Part model, mm, in its own coordinate system. A direction names the side the tool comes from. Give positions to 0.01 mm unless a question says otherwise; leave off trailing zeros. Write each loop counter-clockwise with the first axis right and the second up, starting at its lowest first coordinate (ties: lowest second). Pieces come first, ordered by that corner, then holes.
Autodesk Fusion 360 part; units mm, degrees
sketch "Sketch1" plane through (0, 0, 0) normal (0, 0, 1) x (1, 0, 0)
  line L0 (-50.6234, 49.3431) -> (-3.198, -7.4541)
  line L1 (-2.0113, -7.5) -> (224.0597, -7.5)
  line L2 (-30.2635, 80.5455) -> (225.8084, 7.442)
  line L3 (218.275, -2.7029) -> (218.4394, -2.7498)
  arc A0 (225, -2.55) -> (225, 2.55) centre (225, 0) ccw
  arc A1 (224.0597, -7.5) -> (225.8084, 7.442) centre (224.0646, 0.0728) ccw
  arc A2 (-3.198, -7.4541) -> (-2.0113, -7.5) centre (-2.3159, -0.0062) ccw
  arc A3 (-30.2635, 80.5455) -> (-50.6234, 49.3431) centre (-35.6165, 61.7946) ccw
  circle A4 centre (-35.6165, 61.7946) radius 19.5
  line L4 (55, 15) -> (4.1872, -7.5)
  line L5 (-9.5564, 74.634) -> (40, 40)
  line L6 (-10.2571, 1) -> (-10.2571, 29.4154)
  line L7 (-10.2571, 29.4154) -> (-41.41, 38.3089)
  circle A5 centre (220, 0) radius 2.65
  circle A6 centre (-2.3159, -0.0062) radius 2.65
  circle A7 centre (-35.6165, 61.7946) radius 6.25
  circle A8 centre (-35.6165, 61.7946) radius 18.5
  line L8 (5, 35) -> (20, 35)
  line L9 (20, 35) -> (20, 20)
  line L10 (20, 20) -> (5, 20)
  line L11 (5, 20) -> (5, 35)
  line L12 (130, 20) -> (145, 20)
  line L13 (145, 20) -> (145, 5)
  line L14 (145, 5) -> (130, 5)
  line L15 (130, 5) -> (130, 20)
  circle A9 centre (-20.1665, 61.7946) radius 1.55
  circle A10 centre (-27.8915, 75.1747) radius 1.55
  circle A11 centre (-43.3415, 75.1747) radius 1.55
  circle A12 centre (-51.0665, 61.7946) radius 1.55
  circle A13 centre (-43.3415, 48.4145) radius 1.55
  circle A14 centre (-27.8915, 48.4145) radius 1.55
  circle A15 centre (108.8421, -0.0031) radius 2.65
  line L16 (97.1136, -7.5) -> (55, 15)
  line L17 (150.0703, -7.5) -> (179.7021, 5.621)
  line L18 (179.7021, 5.621) -> (204.2609, -7.5)
  line L19 (40, 40) -> (170.5146, 23.2273)
  circle A16 centre (12.5, 27.5) radius 2.65
  circle A17 centre (137.5, 12.5) radius 2.65
  dimension "d10" = 5.1
  dimension "d44" = 39
  dimension "d49" = 5.3
  dimension "d50" = 5.3
  dimension "d66" = 12.5
  dimension "d67" = 37
  dimension "d114" = 3.1
  dimension "d116" = 360
  dimension "d135" = 5.3
  dimension "d140" = 5.3
  dimension "d141" = 5.3
extrude "Extrude24" add sketch "Sketch1" along normal blind 3 contours L0 L1 L2 A1 A2 A4 L4 L5 L6 L7 L16 L17 L18 L19 | A3 A4 | A8 | L8 L9 L10 L11 | L12 L13 L14 L15 | A16 | A17
extrude "Extrude25" add sketch "Sketch1" along normal blind 21.5 contours L8 L9 L10 L11 | L12 L13 L14 L15 | A16 | A17
extrude "Extrude26" cut sketch "Sketch1" along normal blind 22 contours A16 | A17
fillet "Fillet14" radius 5 1 edges at (-41.41, 38.3089, 1.5)
fillet "Fillet15" radius 10 1 edges at (-10.2571, 29.4154, 1.5)
fillet "Fillet16" radius 5 1 edges at (-10.2571, 1, 1.5)
fillet "Fillet17" radius 10 1 edges at (55, 15, 1.5)
fillet "Fillet18" radius 5 1 edges at (97.1136, -7.5, 1.5)
fillet "Fillet19" radius 5 1 edges at (150.0703, -7.5, 1.5)
fillet "Fillet20" radius 10 1 edges at (179.7021, 5.621, 1.5)
fillet "Fillet21" radius 5 1 edges at (204.2609, -7.5, 1.5)
fillet "Fillet22" radius 10 1 edges at (170.5146, 23.2273, 1.5)
fillet "Fillet23" radius 10 1 edges at (40, 40, 1.5)
fillet "Fillet24" radius 5 1 edges at (-9.5564, 74.634, 1.5)
sketch "Sketch4" plane through (0, 0, 3) normal (0, 0, 1) x (-1, 0, 0)
  arc A0 (8.87, -74.1543) -> (10.3617, -74.8639) centre (11.7343, -70.056) ccw
  line L0 (10.3617, -74.8639) -> (30.2635, -80.5455)
  arc A1 (30.2635, -80.5455) -> (50.6234, -49.3431) centre (35.6165, -61.7946) ccw
  line L1 (50.6234, -49.3431) -> (42.396, -39.4898)
  arc A2 (42.396, -39.4898) -> (39.9306, -37.8866) centre (38.558, -42.6945) ccw
  line L2 (39.9306, -37.8866) -> (17.512, -31.4865)
  arc A3 (10.2571, -21.8707) -> (17.512, -31.4865) centre (20.2571, -21.8707) ccw
  line L3 (10.2571, -21.8707) -> (10.2571, -2.813)
  arc A4 (10.2571, -2.813) -> (9.0951, 0.3917) centre (5.2571, -2.813) ccw
  line L4 (9.0951, 0.3917) -> (3.198, 7.4541)
  arc A5 (3.198, 7.4541) -> (2.0113, 7.5) centre (2.3159, 0.0062) ccw
  line L5 (2.0113, 7.5) -> (-4.1872, 7.5)
  line L6 (-4.1872, 7.5) -> (-50.5405, -13.0253)
  arc A6 (-59.3017, -12.7018) -> (-50.5405, -13.0253) centre (-54.5894, -3.8817) ccw
  line L7 (-59.3017, -12.7018) -> (-96.0094, 6.91)
  arc A7 (-96.0094, 6.91) -> (-98.3655, 7.5) centre (-98.3655, 2.5) ccw
  line L8 (-98.3655, 7.5) -> (-149.0128, 7.5)
  arc A8 (-149.0128, 7.5) -> (-151.0373, 7.0718) centre (-149.0128, 2.5) ccw
  line L9 (-151.0373, 7.0718) -> (-175.2426, -3.6463)
  arc A9 (-184.0038, -3.3228) -> (-175.2426, -3.6463) centre (-179.2915, 5.4973) ccw
  line L10 (-184.0038, -3.3228) -> (-203.1567, 6.91)
  arc A10 (-203.1567, 6.91) -> (-205.5128, 7.5) centre (-205.5128, 2.5) ccw
  line L11 (-205.5128, 7.5) -> (-224.0597, 7.5)
  arc A11 (-224.0597, 7.5) -> (-225.8084, -7.442) centre (-224.0646, -0.0728) ccw
  line L12 (-225.8084, -7.442) -> (-171.2385, -23.0206)
  arc A12 (-171.2385, -23.0206) -> (-169.768, -23.3232) centre (-168.4934, -13.4048) ccw
  line L13 (-169.768, -23.3232) -> (-42.4386, -39.6866)
  arc A13 (-37.9848, -41.4084) -> (-42.4386, -39.6866) centre (-43.7132, -49.605) ccw
  line L14 (-37.9848, -41.4084) -> (8.87, -74.1543)
  line L15 (-5, -20) -> (-5, -35)
  line L16 (-5, -35) -> (-20, -35)
  line L17 (-20, -35) -> (-20, -20)
  line L18 (-20, -20) -> (-5, -20)
  line L19 (-130, -5) -> (-130, -20)
  line L20 (-130, -20) -> (-145, -20)
  line L21 (-145, -20) -> (-145, -5)
  line L22 (-145, -5) -> (-130, -5)
  circle A14 centre (35.6165, -61.7946) radius 6.25
  circle A15 centre (2.3159, 0.0062) radius 2.65
  circle A16 centre (20.1665, -61.7946) radius 1.55
  circle A17 centre (43.3415, -48.4145) radius 1.55
  circle A18 centre (27.8915, -75.1747) radius 1.55
  circle A19 centre (43.3415, -75.1747) radius 1.55
  circle A20 centre (51.0665, -61.7946) radius 1.55
  circle A21 centre (-220, 0) radius 2.65
  circle A22 centre (27.8915, -48.4145) radius 1.55
  circle A23 centre (-108.8421, 0.0031) radius 2.65
  line L23 (-155, -20) -> (-195, -10)
  line L24 (-195, -10) -> (-193.7855, -5.142)
  line L25 (-193.7855, -5.142) -> (-154.3536, -15)
  line L26 (-154.3536, -15) -> (-155, -20)
  line L27 (-30, -25) -> (-110, -25)
  line L28 (-110, -25) -> (-110, -20)
  line L29 (-110, -20) -> (-30, -20)
  line L30 (-30, -20) -> (-30, -25)
  line L31 (-85, -15) -> (-91.3581, -0.6413)
  line L32 (-91.3581, -0.6413) -> (-96.149, -2.7627)
  line L33 (-96.149, -2.7627) -> (-90.238, -16.1118)
  line L34 (-90.238, -16.1118) -> (-89.4127, -20)
  line L35 (-85, -15) -> (-82.786, -20)
  line L36 (5, -65) -> (-20, -44.6537)
  line L37 (-20, -44.6537) -> (-16.1568, -39.9315)
  line L38 (-16.1568, -39.9315) -> (8.0754, -59.653)
  line L39 (8.0754, -59.653) -> (5, -65)
  line L40 (21.4667, -42.2926) -> (3.0133, -20.8693)
  line L41 (3.0133, -20.8693) -> (-1.2182, -24.5142)
  line L42 (-1.2182, -24.5142) -> (16.473, -45.0526)
  line L43 (16.473, -45.0526) -> (21.4667, -42.2926)
extrude "Extrude27" add sketch "Sketch4" along normal blind 1 contours L23 L24 L25 L26 | L27 L28 L29 L30 | L29 L31 L32 L33 L34 L35 | L36 L37 L38 L39 | L40 L41 L42 L43
1) Flat gauge pins, fed straight in: P1, Ø4, axis at x = 148.5, z = 18.5, coming from the -Y side; P2, Ø3.5, axis at x = 211, z = 1.5, coming from the -Y side; P3, Ø19.5, axis at x = 88, y = 8, coming from the +Z side; P4, Ø4.5, axis at x = 9, z = 12.5, coming from the +Y side. Where does each tip first touch, or does it go through?
Check result:
P1: passes through
P2: stops at y = -7.5
P3: stops at z = 4
P4: stops at y = 35
2) Drill centre lines: L1, parallel to Y at x = 137.5, z = 9.5; L2, parallel to Z at x = 47, y = 12; L3, parallel to X at y = 23, z = 14. Where is each one in solid material? Low to high.
Check result:
L1: y = 5 to 9.85, 15.15 to 20
L2: z = 0 to 3
L3: x = 5 to 20
3) Mould opens along X. For faces 6 (the flat face through (138, 5, 12)), 7 (the flat face through (162.97, -1.79, 1.48)), 8 (the flat face through (174.72, 15.07, 3.49)) say: +X half, -X half, draft (parallel to the pull), parting line (faces both ways), or undercut.
Check result:
face 6: draft
face 7: undercut
face 8: +X half
4) 3-axis set-ups, long thin cutter, end or side, ignore diameter. For faces 1 (the flat face through (6, 51, 4)), 2 (the flat face through (27.688, 2.906, 1.479)), 3 (the flat face through (-12.37, 31.73, 3.49)), 4 (the flat face through (93.235, 9.344, 3.493)), 5 (the flat face through (76, 21, 4)): which of +Z, -Z, +X, -X, +Y, -Y reach the whole face in a straight line?
Check result:
face 1: +Z, +X, -X, +Y
face 2: +Z, -Z, -Y
face 3: +Z, -X, -Y
face 4: +Z
face 5: +Z, +Y, -Y
5) Saw through at A-A (x = 220). Write the cut outline in (y, z).
Check result:
outline: (-7.5, 0) - (-2.65, 0) - (-2.65, 3) - (-7.5, 3) - close; (2.65, 0) - (9.1, 0) - (9.1, 3) - (2.65, 3) - close
6) Saw through at C-C (x = 102.5). Write the cut outline in (y, z), and give its area (3 significant figures).
Check result:
outline: (-7.5, 0) - (31.97, 0) - (31.97, 3) - (25, 3) - (25, 4) - (20, 4) - (20, 3) - (-7.5, 3) - close
area: 123 mm2
7) Saw through at B-B (y = 27.5). Write the cut outline in (x, z), and give its area (3 significant figures).
Check result:
outline: (-11.99, 0) - (9.85, 0) - (9.85, 21.5) - (5, 21.5) - (5, 3) - (-1.35, 3) - (-1.35, 4) - (-8.72, 4) - (-8.72, 3) - (-11.99, 3) - close; (15.15, 0) - (137.27, 0) - (137.27, 3) - (20, 3) - (20, 21.5) - (15.15, 21.5) - close
area: 619 mm2
